Could you check a few things on this model? Use its own coordinates, in mm. A direction names the side the tool comes from. Give positions to 0.01 mm unless a question says otherwise; leave off trailing zeros. Order: outer loops, then holes, each group sorted by start corner. A loop starts at its lowest first (then second) coordinate and runs counter-clockwise, first axis right, second up. Notation, with made-up numbers: (-28, 18) - (-1, 18) arc R20 cw to (-1, 52) - close; hole circle Ø10 at (-10.75, -10.75). An arc over 180 degrees is marked (long way). Put each result on its own line as item: value.
Autodesk Inventor part; units mm, degrees
ref_plane "Work Plane1" through (30, 0, 0) normal (0, -0.5, 0.866) x (1, 0, 0)
ref_plane "YZ Plane" through (0, 0, 0) normal (1, 0, 0) x (0, 1, 0)
ref_plane "XZ Plane" through (0, 0, 0) normal (0, 1, 0) x (-1, 0, 0)
sketch "Sketch1" plane through (0, 0, 0) normal (0, 0, 1) x (1, 0, 0)
  line L0 (-0.5833, 0) -> (35, 0)
  line L1 (35, 0) -> (35, 1.25)
  line L2 (35, 1.25) -> (18, 1.25)
  line L3 (18, 1.25) -> (17.7239, 1.25)
  line L4 (17.7239, 1.25) -> (0, 1.25)
  line L5 (0, 1.25) -> (0, 2.25)
  line L6 (0, 2.25) -> (-2.5, 2.25)
  line L7 (-2.5, 2.25) -> (-2.5, 1.1547)
  line L8 (-2.5, 1.1547) -> (-1.25, 1.1547)
  line L9 (-1.25, 1.1547) -> (-0.5833, 0)
  line L10 (-10, 0) -> (42.5, 0)
  line L11 (0, -0.45) -> (0, 2.7)
  line L12 (18, 1.25) -> (0, 1.25) construction
  dimension "d0" = 17
  dimension "d1" = 0.2761
  dimension "d2" = 2.5
  dimension "d3" = 1.25
  dimension "d4" = 60
  dimension "d5" = 2.5
  dimension "d6" = 2.5
  dimension "d7" = 2.3094
  dimension "d8" = 4.5
  dimension "d19" = 35
revolve "Body" add sketch "Sketch1" angle 360 about axis through (-0.5833, 0, 0) along (1, 0, 0)
sketch "Sketch2" plane through (-2.5, 0, 0) normal (-1, 0, 0) x (0, 0, 1)
  circle A0 centre (0, 0) radius 1.1547
  line L0 (0, -3.15) -> (0, 3.15)
  line L1 (-3.15, 0) -> (3.15, 0)
  line L2 (1.1547, 0) -> (0.5774, -1)
  line L3 (0.5774, -1) -> (-0.5774, -1)
  line L4 (-0.5774, -1) -> (-1.1547, 0)
  line L5 (-1.1547, 0) -> (-0.5774, 1)
  line L6 (-0.5774, 1) -> (0.5774, 1)
  line L7 (0.5774, 1) -> (1.1547, 0)
extrude "Slot" add sketch "Sketch2" against normal up to next contours L7 A0 | A0 L2 | L6 L0 A0 | A0 L0 L3 | L0 L6 A0 | A0 L3 L0 | L4 A0 | A0 L5
fillet "Fillet2" radius 0.25 1 edges at (-2.5, -2.25, 0)
thread "Thread"
chamfer "Chamfer1" distance 0.2761 distance2 0.2761 1 edges at (35, -1.25, 0) measured on face at (35, -0.9652, -0.0666)
fillet "Fillet1" radius 0.1 1 edges at (0, -1.25, 0)
ref_plane "Work Plane1" through (30, 0, 0) normal (0, -0.5, 0.866) x (1, 0, 0)
equation "\"d0\" = GEL"
equation "\"d1\" = GAL"
equation "\"d2\" = KOH"
equation "\"d3\" = INTI"
equation "\"d5\" = GD"
equation "\"d6\" = BDM"
equation "\"d7\" = 1.1547 * SW"
equation "\"d8\" = KOD"
equation "\"d19\" = NLG"
equation "\"d16\" = RR"
equation "\"d12\" = GEL"
equation "\"d14\" = -0.5 * SPD + 0.5 * GD"
equation "\"d15\" = GUL"
equation "\"d29\" = R"
equation "\"GD\" = NND"
equation "\"NLG\" = 35"
equation "\"GEL\" = 17"
equation "\"KOD\" = 4.5"
equation "\"KOH\" = 2.5"
equation "\"INTI\" = 1.25"
equation "\"GAL\" = 0.61345 * PTC"
equation "\"GUL\" = 0.61345 * PTC"
equation "\"BDM\" = NND"
equation "\"SW\" = 2"
equation "\"RR\" = 0.25"
equation "\"SPD\" = 1.94789"
equation "\"d28\" = R"
equation "\"R\" = 0.1"
equation "\"TOA\" = 30deg"
equation "\"THREADDIA\" = 2.5"
equation "\"KOD1\" = KOD"
equation "\"PTC\" = 0.45"
equation "\"NND\" = 2.5"
equation "\"E0\" = 1.155 * SW"
equation "\"GD1\" = THREADDIA - 1.2269 * PTC"
properties part number "ANSI B18.3.1M - M2,5x0,45 x 35" material "Steel, Mild"
1) We'd pull the mould along Z, two halves only. Please class faces 1 (the flat face through (0, 0.5, -1.5)), 2 (the flat face through (-1.84, 0.49, -0.87)), 3 (the cylindrical face through (17.17, -0.27, 1.22)): pulls with the +Z half, pulls with the -Z half, needs draft (parallel to the pull), parting line crosses it, or undercut.
Filled in:
face 1: needs draft
face 2: undercut
face 3: parting line crosses it
2) Suppose I cut it at A-A, the plane x = 23.5. List the corners of the cut face in (y, z) for me.
Filled in:
outline: circle Ø2.5 at (0, 0)
3) If I drill on line 1 (Z direction, x = 11, y = -0.1); line 2 (X direction, y = -0.15, z = 1.45), over which ranges is the centre line in solid material (lowest first)? Write a range as [from, to].
Filled in:
line 1: z = [-1.25, 1.25]
line 2: x = [-2.5, 0]
4) I'm going to push flat-ended pins straight in: pin 1 (2 mm diameter, centred on x = 6.5, z = 0.5, fed in from -Y); pin 2 (1 mm diameter, centred on x = 25.5, y = -0.5, fed in from -Z). Where does each tip first touch, or does it pass through?
Filled in:
pin 1: stops at y = -1.25
pin 2: stops at z = -1.25
5) Which directions (+Z, -Z, +X, -X, +Y, -Y) give clear straight access to the entire face, cutting with the end or side of a thin tool? Please do faces 4 (the flat face through (-2, -1, 0)), 5 (the cylindrical face through (-1.14, -0.29, -2.23)).
Filled in:
face 4: -X
face 5: +X, -X
